For this review, take the finished solid that the model builds, in its own axes (mm). A direction names the side the tool comes from. Round coordinates to 2 decimals unless told otherwise and drop trailing zeros. Loops run counter-clockwise (first coordinate to the right, second up) from the corner with the lowest first, then second, coordinate; pieces in that order, holes last.
1. To check wall thickness, follow line 1 along X through (y, z) = (3.5, -0.4); line 2 along Z through (x, y) = (-3.5, 6.75); line 3 along Z through (x, y) = (-3, 5). State the ranges of each line that lie inside material, in increasing order.
2. Consider section A-A on z = 1.2. State the section outline as (x, y) points, then the cut area to 3 significant figures.
3. Consider section C-C on y = 2.75. State the section outline as (x, z) points.
4. Clearance check with flat-ended pins moving along their axes: pin 1 Ø1.6 at (x, y) = (1, 1) entering from +Z; pin 2 Ø0.5 at (x, y) = (1.5, 7.5) entering from +Z; pin 3 Ø0.8 at (y, z) = (3.5, -1.5) entering from -X. State where each tip first meets the part, or that it passes through.
5. Tool access review of faces 1 (the flat face through (0, 1, 2)), 2 (the flat face through (-4.5, 1, 0)), 3 (the flat face through (-4, 4.5, -1.5)), 4 (the flat face through (-3.5, 5.5, -2.5)): name each direction out of +Z, -Z, +X, -X, +Y, -Y from which nothing blocks a thin tool from reaching the whole face with its end or side.
6. Consider section D-D on x = -3.75. State the section outline as (y, z) points, then the cut area to 4 significant figures.
7. Consider section B-B on x = -1.75. State the section outline as (y, z) points.
from build123d import *

# Parameters (mm, degrees)
SKETCH1_W           = 8
SKETCH1_H           = 6
BOSS_EXTRUDE1_DEPTH = 8
SKETCH2_W           = 1
SKETCH2_H           = 2
CUT_EXTRUDE1_DEPTH  = 9
SKETCH3_W           = 7
SKETCH3_H           = 4
CUT_EXTRUDE2_DEPTH  = 1
SKETCH4_W           = 3
SKETCH4_H           = 1
CUT_EXTRUDE3_DEPTH  = 2
CUT_EXTRUDE4_DEPTH  = 3
SKETCH8_W           = 1
SKETCH8_H           = 1
CUT_EXTRUDE7_DEPTH  = 1
CUT_EXTRUDE8_DEPTH  = 3
CUT_EXTRUDE9_DEPTH  = 1
SKETCH14_W          = 4
SKETCH14_H          = 2
CUT_EXTRUDE12_DEPTH = 1
BOSS_EXTRUDE2_DEPTH = 1
SKETCH16_W          = 1
SKETCH16_H          = 1
CUT_EXTRUDE13_DEPTH = 5
CUT_EXTRUDE14_DEPTH = 1


with BuildPart() as part:
    # Sketch1 → Boss-Extrude1 (new body)
    with BuildSketch(Plane(origin=(0, 0, 0), x_dir=(1, 0, 0), z_dir=(0, 1, 0))):
        Rectangle(SKETCH1_W, SKETCH1_H)
    extrude(amount=BOSS_EXTRUDE1_DEPTH)

    # Sketch2 → Cut-Extrude1 (cut, through all)
    with BuildSketch(Plane.ZY.offset(4)):
        with Locations((2.5, 1)):
            Rectangle(SKETCH2_W, SKETCH2_H)
    extrude(amount=-CUT_EXTRUDE1_DEPTH, mode=Mode.SUBTRACT)

    # Sketch3 → Cut-Extrude2 (cut)
    with BuildSketch(Plane.XY.offset(3)):
        with Locations((-0.5, 6)):
            Rectangle(SKETCH3_W, SKETCH3_H)
    extrude(amount=-CUT_EXTRUDE2_DEPTH, mode=Mode.SUBTRACT)

    # Sketch4 → Cut-Extrude3 (cut)
    with BuildSketch(Plane.XY.offset(3)):
        with Locations((2.5, 7.5)):
            Rectangle(SKETCH4_W, SKETCH4_H)
    extrude(amount=-CUT_EXTRUDE3_DEPTH, mode=Mode.SUBTRACT)

    # Sketch5 → Cut-Extrude4 (cut)
    with BuildSketch(Plane.XY.offset(2)):
        Polygon((1, 8), (-3, 4), (-4, 4), (-4, 8), align=None)
    extrude(amount=-CUT_EXTRUDE4_DEPTH, mode=Mode.SUBTRACT)

    # Sketch8 → Cut-Extrude7 (cut)
    with BuildSketch(Plane(origin=(1, 0, 0), x_dir=(0, 0, -1), z_dir=(1, 0, 0))):
        with Locations((-1.5, 7.5)):
            Rectangle(SKETCH8_W, SKETCH8_H)
    extrude(amount=-CUT_EXTRUDE7_DEPTH, mode=Mode.SUBTRACT)

    # Sketch9 → Cut-Extrude8 (cut, through all)
    with BuildSketch(Plane.XY.offset(-1)):
        Polygon((0, 8), (1, 8), (0, 7), align=None)
    extrude(amount=-CUT_EXTRUDE8_DEPTH, mode=Mode.SUBTRACT)

    # Sketch10 → Cut-Extrude9 (cut)
    with BuildSketch(Plane(origin=(0, 8, 0), x_dir=(1, 0, 0), z_dir=(0, 1, 0))):
        Polygon((-4, 1), (-4, 2), (-2, 2), (-2, 3), (0, 3), (0, 1), align=None)
    extrude(amount=-CUT_EXTRUDE9_DEPTH, mode=Mode.SUBTRACT)

    # Sketch14 → Cut-Extrude12 (cut)
    with BuildSketch(Plane.ZY.offset(4)):
        with Locations((1, 3)):
            Rectangle(SKETCH14_W, SKETCH14_H)
    extrude(amount=-CUT_EXTRUDE12_DEPTH, mode=Mode.SUBTRACT)

    # Sketch15 → Boss-Extrude2 (add)
    with BuildSketch(Plane.ZY.offset(4)):
        Polygon((-3, 8), (-2, 8), (-2, 7), (-1, 7), (-1, 2), (0, 2), (0, 0), (-3, 0), align=None)
    extrude(amount=BOSS_EXTRUDE2_DEPTH)

    # Sketch16 → Cut-Extrude13 (cut)
    with BuildSketch(Plane(origin=(0, 7, 0), x_dir=(1, 0, 0), z_dir=(0, 1, 0))):
        with Locations((-4.5, 1.5)):
            Rectangle(SKETCH16_W, SKETCH16_H)
    extrude(amount=-CUT_EXTRUDE13_DEPTH, mode=Mode.SUBTRACT)

    # Sketch17 → Cut-Extrude14 (cut)
    with BuildSketch(Plane(origin=(0, 0, -3), x_dir=(-1, 0, 0), z_dir=(0, 0, -1))):
        Polygon((2, 7), (5, 4), (5, 8), (2, 8), align=None)
    extrude(amount=-CUT_EXTRUDE14_DEPTH, mode=Mode.SUBTRACT)


solid = part.part
Resolved:
1. line 1: x = -3 to 4
1. line 2: z = -2 to -1
1. line 3: z = -3 to -1
2. outline: (-4, 0) - (4, 0) - (4, 7) - (0, 7) - (-3, 4) - (-3, 2) - (-4, 2) - close
2. area: 46.5 mm2
3. outline: (-5, -3) - (4, -3) - (4, 3) - (-3, 3) - (-3, -1) - (-4, -1) - (-4, -2) - (-5, -2) - close
4. pin 1: stops at z = 2
4. pin 2: stops at z = 1
4. pin 3: stops at x = -4
5. face 1: +Z, +X, -X, -Y
5. face 2: +Z, -X, +Y, -Y
5. face 3: +Z, -X, +Y
5. face 4: -Z, -X, +Y
6. outline: (0, -3) - (5.25, -3) - (5.25, -2) - (7, -2) - (7, -1) - (2, -1) - (2, 2) - (0, 2) - close
6. area: 18.25 mm2
7. outline: (0, -3) - (7, -3) - (7, -1) - (5.25, -1) - (5.25, 2) - (4, 2) - (4, 3) - (2, 3) - (2, 2) - (0, 2) - close
